The listing builds one solid part. Answer for the finished solid, in the listing's coordinates (mm). A direction names the side the tool comes from. Give positions to 0.01 mm unless a question says otherwise; leave off trailing zeros. Order: outer loops, then holes, each group sorted by start corner. A loop starts at its lowest first (then second) coordinate and runs counter-clockwise, first axis right, second up. Notation, with made-up numbers: (26, 35) - (63, 35) arc R12 cw to (63, 39) - close; hole circle Ø5 at (26.25, -22). An arc over 180 degrees is marked (long way). Write each question's results on one line, items separated by ' | '. Start each with the question number.
1. Which of the six approach directions +Z, -Z, +X, -X, +Y, -Y give full straight-line access (tool end or side, diameter ignored) to faces 1 (the face through (19.05, 11, 0)), 2 (the face through (59, 50, -6.35)), 3 (the face through (-6.35, 61.03, -0.14))?
2. Flat-ended cylindrical pins translate along their axes: pin 1 (10 mm diameter, centred on x = 2, z = 0, fed in from -Y); pin 2 (6 mm diameter, centred on y = 56.5, z = 1.5, fed in from +X); pin 3 (1 mm diameter, centred on y = 21.5, z = -1.5, fed in from +X). Find the tip coordinate at first contact, or state that the pin passes through.
3. Section D-D (z = -15) is taken. Give the vertices of the cut face in (x, y).
4. Find the intervals of material crossed by L1, parallel to Z at x = 0, y = 39; L2, parallel to Z at x = 31, y = 92.5, in increasing order.
5. Section C-C (x = 48) is taken. Give the vertices of the cut face in (y, z), and give its area (3 significant figures).
6. Section A-A (y = 47) is taken. Give the vertices of the cut face in (x, z) (3 decimals), and give its area (3 significant figures).
7. Determine the mould class of faces 4 (the face through (77, 0, -2)), 5 (the face through (0.99, 61.03, 3.15)), 6 (the face through (133.47, 50.089, -21.926)), 7 (the face through (59, 50, 6.35)) for opening direction Z: released by +Z, released by -Z, zero draft, split by the parting line, or undercut.
8. Section B-B (z = 0) is taken. Give the vertices of the cut face in (x, y).
from build123d import *

# Parameters (mm, degrees)
SKETCH1_R           = 3.302
BOSS_EXTRUDE1_DEPTH = 101.6
SKETCH2_W           = 25.4
SKETCH2_H           = 21.59
CUT_EXTRUDE1_DEPTH  = 173.667733558


with BuildPart() as part:
    # Sketch1 → Boss-Extrude1 (new body)
    # profile 1 of 3: a face of its own
    with BuildSketch(Plane(origin=(0, 0, 0), x_dir=(1, 0, 0), z_dir=(0, 1, 0))):
        with BuildLine():
            Line((116.983825791, 6.35), (0, 6.35))
            ThreePointArc((0, 6.35), (-6.35, 0), (0, -6.35))
            Line((0, -6.35), (120.65, -6.35))
            ThreePointArc((120.65, -6.35), (115.150738686, -3.175), (115.150738686, 3.175))
            Line((115.150738686, 3.175), (116.983825791, 6.35))
        make_face()
        with Locations(Location((0, 0, 0), (0, 0, 270))):
            Circle(SKETCH1_R, mode=Mode.SUBTRACT)
    # profile 2 of 3: a face of its own
    with BuildSketch(Plane(origin=(0, 0, 0), x_dir=(1, 0, 0), z_dir=(0, 1, 0))):
        with BuildLine():
            Line((120.65, 6.35), (116.983825791, 6.35))
            Line((116.983825791, 6.35), (115.150738686, 3.175))
            ThreePointArc((115.150738686, 3.175), (115.150738686, -3.175), (120.65, -6.35))
            ThreePointArc((120.65, -6.35), (123.825, -5.499261314), (126.149261314, -3.175))
            ThreePointArc((126.149261314, -3.175), (126.149261314, 3.175), (120.65, 6.35))
        make_face()
    # profile 3 of 3: a face of its own
    with BuildSketch(Plane(origin=(0, 0, 0), x_dir=(1, 0, 0), z_dir=(0, 1, 0))):
        with BuildLine():
            Line((124.675738686, 19.672783942), (116.983825791, 6.35))
            Line((116.983825791, 6.35), (120.65, 6.35))
            ThreePointArc((120.65, 6.35), (126.149261314, 3.175), (126.149261314, -3.175))
            Line((126.149261314, -3.175), (135.674261314, 13.322783942))
            ThreePointArc((135.674261314, 13.322783942), (133.35, 21.997045256), (124.675738686, 19.672783942))
        make_face()
    extrude(amount=BOSS_EXTRUDE1_DEPTH)

    # Sketch2 → Cut-Extrude1 (cut, through all)
    with BuildSketch(Plane.XY.offset(6.35)):
        with Locations((6.35, 10.795)):
            Rectangle(SKETCH2_W, SKETCH2_H)
    extrude(amount=-CUT_EXTRUDE1_DEPTH, mode=Mode.SUBTRACT)


solid = part.part
Reported:
1) face 1: +Z, -Z, -X, -Y | face 2: -Z, -X, +Y, -Y | face 3: -X, +Y, -Y
2) pin 1: y = 21.59 | pin 2: x = 128.85 | pin 3: x = 129.14
3) outline: (121.98, 0) - (136.35, 0) - (136.35, 101.6) - (121.98, 101.6) - close
4) L1: -6.35 to -3.3, 3.3 to 6.35 | L2: -6.35 to 6.35
5) outline: (0, -6.35) - (101.6, -6.35) - (101.6, 6.35) - (0, 6.35) - close | area: 1,290 mm²
6) outline: (0, -6.35) - (116.984, -6.35) - (124.676, -19.673) arc R6.35 ccw to (135.674, -13.323) - (126.149, 3.175) arc R6.35 ccw to (120.65, 6.35) - (0, 6.35) arc R6.35 ccw to start; hole circle Ø6.604 at (0, 0) | area: 1,860 mm²
7) face 4: zero draft | face 5: undercut | face 6: split by the parting line | face 7: released by +Z
8) outline: (-6.35, 21.59) - (-3.3, 21.59) - (-3.3, 101.6) - (-6.35, 101.6) - close; (3.3, 21.59) - (19.05, 21.59) - (19.05, 0) - (127.98, 0) - (127.98, 101.6) - (3.3, 101.6) - close
